```python
from build123d import *

# Parameters (mm, degrees)
SKETCH003_W      = 38.1
SKETCH003_H      = 31.75
PAD002_DEPTH     = 2.54
SKETCH004_R      = 3.175
PAD003_DEPTH     = 15.24
SKETCH005_R      = 5.08
POCKET001_DEPTH  = 17.781
SKETCH006_R      = 6.604
PAD004_DEPTH     = 9.525
SKETCH007_W      = 6.35
SKETCH007_H      = 35.56
SKETCH007_R      = 1.2065
PAD005_DEPTH     = 2.54
SKETCH008_W      = 3.175
SKETCH008_H      = 15.24
PAD006_DEPTH     = 3.81
POCKET002_DEPTH  = 15.24
SKETCH010_W      = 15.24
SKETCH010_H      = 2.54
PAD007_DEPTH     = 2.54
CHAMFER_ANGLE    = 25
CHAMFER_SIZE     = 3.81
SKETCH011_R      = 3.683
POCKET003_DEPTH  = 2.541
POCKET004_DEPTH  = 0.508
HOLE_D           = 2.54
HOLE_CBORE_D     = 5.715
HOLE_CBORE_DEPTH = 1.27
SKETCH014_R      = 1.016
POCKET005_DEPTH  = 12.7
CHAMFER001_SIZE  = 1.524


with BuildPart() as part:
    # Sketch003 → Pad002 (new body)
    with BuildSketch(Plane.XZ):
        with BuildLine():
            ThreePointArc((-50.8, -20), (-47.080256, -28.980256), (-38.1, -32.7))
            Line((111.9, -32.7), (-38.1, -32.7))
            ThreePointArc((111.9, -32.7), (120.880256, -28.980256), (124.6, -20))
            Line((124.6, 20), (124.6, -20))
            ThreePointArc((124.6, 20), (120.880256, 28.980256), (111.9, 32.7))
            Line((-38.1, 32.7), (111.9, 32.7))
            ThreePointArc((-38.1, 32.7), (-47.080256, 28.980256), (-50.8, 20))
            Line((-50.8, -20), (-50.8, 20))
        make_face()
        Rectangle(SKETCH003_W, SKETCH003_H, mode=Mode.SUBTRACT)
    extrude(amount=PAD002_DEPTH)

    # Sketch004 (on Face13 of Pad002) → Pad003 (join)
    with BuildSketch(Plane(origin=(0, 0, 0), x_dir=(1, 0, 0), z_dir=(0, 1, 0))):
        with Locations((111.9, -20)):
            Circle(SKETCH004_R)
        with Locations((111.9, 20)):
            Circle(SKETCH004_R)
        with Locations((-38.1, -20)):
            Circle(SKETCH004_R)
        with Locations((-38.1, 20)):
            Circle(SKETCH004_R)
        with Locations((36.9, 20)):
            Circle(SKETCH004_R)
        with Locations((36.9, -20)):
            Circle(SKETCH004_R)
    extrude(amount=PAD003_DEPTH)

    # Sketch005 (on Face5 of Pad003) → Pocket001 (cut, through all)
    with BuildSketch(Plane.XZ.offset(2.54)):
        with Locations((90.293198, 5.763262)):
            Circle(SKETCH005_R)
        with Locations((74.627113, 5.763262)):
            Circle(SKETCH005_R)
    extrude(amount=-POCKET001_DEPTH, mode=Mode.SUBTRACT)

    # Sketch006 (on Face4 of Pocket001) → Pad004 (join)
    with BuildSketch(Plane(origin=(0, 0, 0), x_dir=(1, 0, 0), z_dir=(0, 1, 0))):
        with BuildLine():
            ThreePointArc((74.627113, 3.126738), (65.737113, -5.763262), (74.627113, -14.653262))
            Line((90.293198, -14.653262), (74.627113, -14.653262))
            ThreePointArc((90.293198, -14.653262), (99.183198, -5.763262), (90.293198, 3.126738))
            Line((74.627113, 3.126738), (90.293198, 3.126738))
        make_face()
        with Locations((90.293198, -5.763262)):
            Circle(SKETCH006_R, mode=Mode.SUBTRACT)
        with Locations((74.627113, -5.763262)):
            Circle(SKETCH006_R, mode=Mode.SUBTRACT)
    extrude(amount=PAD004_DEPTH)

    # Sketch007 (on Face4 of Pad004) → Pad005 (join)
    with BuildSketch(Plane(origin=(0, 0, 0), x_dir=(1, 0, 0), z_dir=(0, 1, 0))):
        with Locations((23.622, 0)):
            Rectangle(SKETCH007_W, SKETCH007_H)
        with Locations((22.479, 14.605)):
            Circle(SKETCH007_R, mode=Mode.SUBTRACT)
        with Locations((22.479, -14.605)):
            Circle(SKETCH007_R, mode=Mode.SUBTRACT)
        with Locations((-29.718, 0)):
            Rectangle(SKETCH007_W, SKETCH007_H)
        with Locations((-28.321, -14.605)):
            Circle(SKETCH007_R, mode=Mode.SUBTRACT)
        with Locations((-28.321, 14.605)):
            Circle(SKETCH007_R, mode=Mode.SUBTRACT)
    extrude(amount=PAD005_DEPTH)

    # Sketch008 (on Face37 of Pad005) → Pad006 (join)
    with BuildSketch(Plane(origin=(0, 2.54, 0), x_dir=(1, 0, 0), z_dir=(0, 1, 0))):
        with Locations((25.2095, 0)):
            Rectangle(SKETCH008_W, SKETCH008_H)
        with Locations((-31.3055, 0)):
            Rectangle(SKETCH008_W, SKETCH008_H)
    extrude(amount=PAD006_DEPTH)

    # Sketch009 (on Face54 of Pad006) → Pocket002 (cut)
    with BuildSketch(Plane(origin=(0, 0, -7.62), x_dir=(1, 0, 0), z_dir=(0, 0, -1))):
        Polygon((23.622, -2.54), (25.146, -2.54), (25.146, -4.318), (24.003, -4.318), (25.146, -6.35), (23.622, -6.35), align=None)
        Polygon((-29.718, -2.54), (-31.242, -2.54), (-31.242, -4.318), (-30.099, -4.318), (-31.242, -6.35), (-29.718, -6.35), align=None)
    extrude(amount=-POCKET002_DEPTH, mode=Mode.SUBTRACT)

    # Sketch010 (on Face4 of Pocket002) → Pad007 (join)
    with BuildSketch(Plane(origin=(0, 0, 0), x_dir=(1, 0, 0), z_dir=(0, 1, 0))):
        with Locations((0, -19.05)):
            Rectangle(SKETCH010_W, SKETCH010_H)
    extrude(amount=PAD007_DEPTH)

    # Chamfer
    chamfer_edges = [part.edges().sort_by_distance(p)[0] for p in [
        (0, -2.54, -15.875),
        (19.05, -2.54, 0),
        (0, -2.54, 15.875),
        (-19.05, -2.54, 0),
    ]]
    chamfer_side = part.faces().sort_by_distance((40.639586, -2.54, -0.093816))[0]
    chamfer(chamfer_edges, length=CHAMFER_SIZE, angle=CHAMFER_ANGLE, reference=chamfer_side)

    # Sketch011 (on Face20 of Chamfer) → Pocket003 (cut, through all)
    with BuildSketch(Plane(origin=(0, 0, 0), x_dir=(1, 0, 0), z_dir=(0, 1, 0))):
        with Locations((95.99, 13.286738)):
            Circle(SKETCH011_R)
        with Locations((74.4, 13.286738)):
            Circle(SKETCH011_R)
        with Locations((52.81, 13.286738)):
            Circle(SKETCH011_R)
    extrude(amount=-POCKET003_DEPTH, mode=Mode.SUBTRACT)

    # Sketch012 (on Face1 of Pocket003) → Pocket004 (cut)
    with BuildSketch(Plane.XZ.offset(2.54)):
        Polygon((49.803737, -8.079738), (55.816263, -8.079738), (58.822526, -13.286738), (55.816263, -18.493738), (49.803737, -18.493738), (46.797474, -13.286738), align=None)
        Polygon((71.393737, -8.079738), (77.406263, -8.079738), (80.412526, -13.286738), (77.406263, -18.493738), (71.393737, -18.493738), (68.387474, -13.286738), align=None)
        Polygon((92.983737, -8.079738), (98.996263, -8.079738), (102.002526, -13.286738), (98.996263, -18.493738), (92.983737, -18.493738), (89.977474, -13.286738), align=None)
    extrude(amount=-POCKET004_DEPTH, mode=Mode.SUBTRACT)

    # Hole (through all)
    with Locations(Plane.XZ.offset(2.54)):
        with Locations((119.52, 17.78), (119.52, -17.78), (-45.72, -17.78), (-45.72, 17.78)):
            CounterBoreHole(HOLE_D / 2, HOLE_CBORE_D / 2, HOLE_CBORE_DEPTH)

    # Sketch014 (on Face90 of Hole) → Pocket005 (cut)
    with BuildSketch(Plane(origin=(0, 15.24, 0), x_dir=(1, 0, 0), z_dir=(0, 1, 0))):
        with Locations((-38.1, 20)):
            Circle(SKETCH014_R)
        with Locations((-38.1, -20)):
            Circle(SKETCH014_R)
        with Locations((36.9, -20)):
            Circle(SKETCH014_R)
        with Locations((36.9, 20)):
            Circle(SKETCH014_R)
        with Locations((111.9, 20)):
            Circle(SKETCH014_R)
        with Locations((111.9, -20)):
            Circle(SKETCH014_R)
    extrude(amount=-POCKET005_DEPTH, mode=Mode.SUBTRACT)

    # Chamfer001
    chamfer001_edges = [part.edges().sort_by_distance(p)[0] for p in [
        (-41.275, 0, -20),
        (-41.275, 0, 20),
        (33.725, 0, 20),
        (33.725, 0, -20),
        (108.725, 0, 20),
        (108.725, 0, -20),
    ]]
    chamfer(chamfer001_edges, length=CHAMFER001_SIZE)


solid = part.part
```
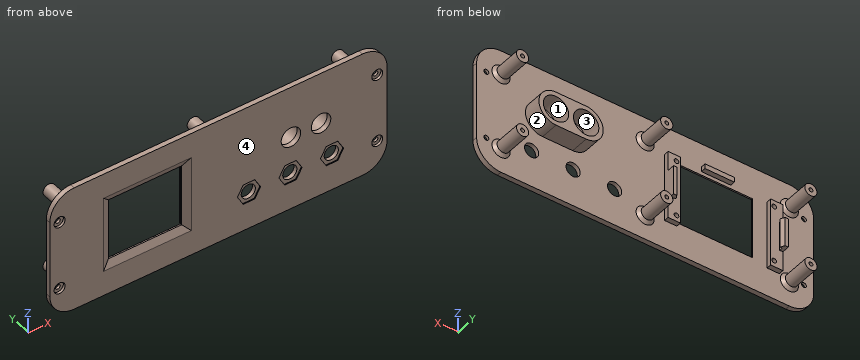
Work out the finished part from the listing and answer in its coordinate system (mm). Face numbers are marked on the shaded views. Give positions to 0.01 mm unless a question says otherwise; leave off trailing zeros. Use CSV: the item, a comma, the result in double quotes. Start each with the question number.
(1) Find section A-A, the plane y = 13.5. Count the separate pieces of the cut face and the enclosed holes in it, plus the area to 3 significant figures.
(2) Each of these flat-tipped pins is pushed along its axis until it touches: pin 1 (2.5 mm diameter, centred on x = 23, z = -14, fed in from +Y); pin 2 (16.5 mm diameter, centred on x = 90.29, z = 5.76, fed in from +Y) (3 decimals); pin 3 (2 mm diameter, centred on x = -28.321, z = 14.605, fed in from +Y). Where does it stop, or does it pass through?
(3) Determine the mould class of the marked faces 1, 2, 3 and 4 for opening direction Z: released by +Z, released by -Z, zero draft, split by the parting line, or undercut.
(4) Find the intervals of material crossed by L1, parallel to Z at x = 36.9, y = 7 (3 decimals); L2, parallel to Z at x = 74.4, y = -1.6; L3, parallel to X at y = -0.5, z = 0, in increasing order.
Results found:
1,separate pieces,"6"
1,enclosed holes,"6"
1,area,"171 mm^2"
2,pin 1,"y = 2.54"
2,pin 2,"y = 9.525"
2,pin 3,"y = 0"
3,face 1,"undercut"
3,face 2,"split by the parting line"
3,face 3,"undercut"
3,face 4,"zero draft"
4,L1,"-23.175 to -21.016, -18.984 to -16.825, 16.825 to 18.984, 21.016 to 23.175"
4,L2,"-32.7 to -16.97, -9.6 to 0.69, 10.84 to 32.7"
4,L3,"-50.8 to -19.05, 19.05 to 124.6"
